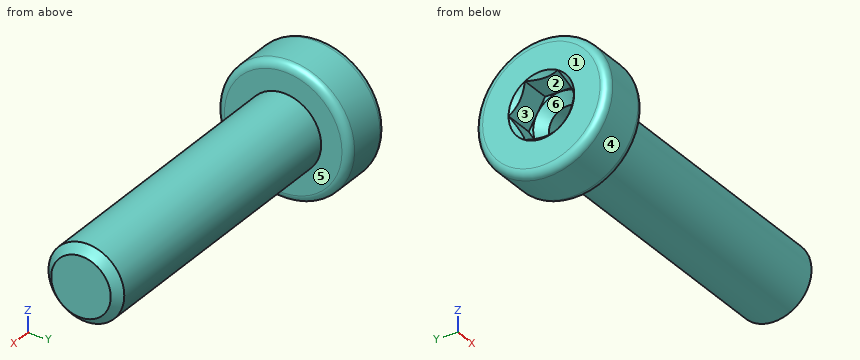
Autodesk Inventor part; units mm, degrees
ref_plane "MONTAGE_XY" through (0, 0, 0) normal (1, 0, 0) x (0, 0, -1)
ref_plane "MONTAGE_YZ" through (0, 0, 0) normal (0, 0, -1) x (0, 1, 0)
ref_plane "MONTAGE_ZX" through (0, 0, 0) normal (0, 1, 0) x (1, 0, 0)
sketch "Sketch_1" plane through (0, 0, 0) normal (0, 0, 1) x (1, 0, 0)
  line L0 (16, 0) -> (1.5, 0)
  line L1 (1.5, 0) -> (0.5, 1)
  line L2 (0.5, 1) -> (-0.7, 1)
  line L3 (-0.7, 1) -> (-1.2, 1.5)
  line L4 (-1.2, 1.5) -> (-2.5679, 1.5)
  line L5 (-2.5679, 1.5) -> (-2.8, 1.7321)
  line L6 (-2.8, 1.7321) -> (-2.8, 3.1)
  arc A0 (-2.4, 3.5) -> (-2.8, 3.1) centre (-2.4, 3.1) ccw
  line L7 (-2.4, 3.5) -> (-0.4, 3.5)
  arc A1 (0, 3.1) -> (-0.4, 3.5) centre (-0.4, 3.1) ccw
  line L8 (0, 3.1) -> (0, 2)
  line L9 (0, 2) -> (15.5705, 2)
  line L10 (15.5705, 2) -> (16, 1.5705)
  line L11 (16, 1.5705) -> (16, 0)
  line L12 (16, 0) -> (1.5, 0)
revolve "Revolution1" add sketch "Sketch_1" angle 360 about axis through (16, 0, 0) along (-1, 0, 0)
thread "Thread1"
sketch "Sketch_2" plane through (-2.8, 0, 0) normal (1, 0, 0) x (0, 0, -1)
  line L0 (-1.5, -0.866) -> (0, -1.7321)
  line L1 (0, -1.7321) -> (1.5, -0.866)
  line L2 (1.5, -0.866) -> (1.5, 0.866)
  line L3 (1.5, 0.866) -> (0, 1.7321)
  line L4 (0, 1.7321) -> (-1.5, 0.866)
  line L5 (-1.5, 0.866) -> (-1.5, -0.866)
extrude "Extrusion1" cut sketch "Sketch_2" along normal blind 1.6
ref_plane "MONTAGE_XY" through (0, 0, 0) normal (1, 0, 0) x (0, 0, -1)
ref_plane "MONTAGE_YZ" through (0, 0, 0) normal (0, 0, -1) x (0, 1, 0)
ref_plane "MONTAGE_ZX" through (0, 0, 0) normal (0, 1, 0) x (1, 0, 0)
ref_plane "Schrauben_punkt_XY" through (16, 0, 0) normal (-1, 0, 0) x (0, 0, -1)
ref_plane "Schrauben_punkt_YZ" through (16, 0, 0) normal (0, 0, -1) x (0, -1, 0)
ref_plane "Schrauben_punkt_ZX" through (16, 0, 0) normal (0, -1, 0) x (-1, 0, 0)
properties part number "DIN-6912 - M4x16(F)"
Here's how the part is built. I have some questions about the finished solid (model axes, mm). Face numbers are marked on the shaded views. A direction names the side the tool comes from. Give positions to 0.01 mm unless a question says otherwise; leave off trailing zeros. Write each loop counter-clockwise with the first axis right and the second up, starting at its lowest first coordinate (ties: lowest second). Pieces come first, ordered by that corner, then holes. Notation, with made-up numbers: (71, -24) -> (119, -24) arc R11 ccw to (119, -17) -> close; hole circle Ø7 at (-36.5, 75). An arc over 180 degrees is marked (long way). Use one line per item in the form item = value.
1) We'd pull the mould along Z, two halves only. Please class the marked faces 1, 2, 3 and 4: +Z half, -Z half, draft (parallel to the pull), parting line (faces both ways), or undercut.
Verdict:
face_1 = draft
face_2 = undercut
face_3 = undercut
face_4 = parting line
2) I'm going to push flat-ended pins straight in: pin 1 (4 mm diameter, centred on x = 10, y = -2, fed in from -Z); pin 2 (1.4 mm diameter, centred on y = -0.5, z = -0.5, fed in from -X); pin 3 (1.8 mm diameter, centred on x = -2, y = 0.5, fed in from -Z); pin 4 (3 mm diameter, centred on x = 9.5, y = -2, fed in from +Z). Where does each tip first touch, or does it pass through?
Verdict:
pin_1 = -2
pin_2 = -1.11
pin_3 = -3.5
pin_4 = 1.94
3) If I drill on L1, parallel to Y at x = 0.2, z = 0; L2, parallel to X at y = 0.75, z = -3, over which ranges is the centre line in solid material (lowest first)? Write a range as [from, to].
Verdict:
L1 = [-2, -1], [1, 2]
L2 = [-2.8, 0]
4) On a 3-axis mill with a long thin cutter (end or side, diameter ignored), from which of +Z, -Z, +X, -X, +Y, -Y can I reach the whole of each face in a straight line? I mean the marked faces 5 and 6. Say none if no direction works.
Verdict:
face_5 = +X
face_6 = -X
5) Suppose I cut it at A-A (x = 5). Please give me the cut outline in (y, z).
Verdict:
outline = circle Ø4 at (0, 0)
